Verification items for the finished model (mm, model axes). Face numbers are marked on the shaded views. Give positions to 0.01 mm unless a question says otherwise; leave off trailing zeros. Write each loop counter-clockwise with the first axis right and the second up, starting at its lowest first coordinate (ties: lowest second). Pieces come first, ordered by that corner, then holes. Notation, with made-up numbers: (-37.75, 1) -> (16.25, 1) arc R21 ccw to (16.25, 26) -> close; hole circle Ø6 at (13.25, 21.25). An arc over 180 degrees is marked (long way). Use one line per item in the form item = value. Start each with the question number.
(1) Section check A-A, the plane y = -50.8. Record the cut outline in (x, z).
(2) Depth check by flat-ended pin: pin 1 Ø2 at (y, z) = (-23, -80) entering from -X; pin 2 Ø10 at (x, y) = (-141, -20.5) entering from +Z; pin 3 Ø12.5 at (x, y) = (169, -68.5) entering from -Z. Enter the tip coordinate at first touch or a pass-through.
(3) Scan lines: L1, parallel to Z at x = -89, y = -24.5; L2, parallel to X at y = -82, z = -135; L3, parallel to X at y = -45, z = 368.5. Record each from-to range of solid material in increasing order.
(4) Section check B-B, the plane z = -79.5. Record the cut outline in (x, y), plus the area to 3 significant figures.
(5) Release check for a two-part mould opening along Z. For the marked faces 1, 2 and 3 record: pulls with the +Z half, pulls with the -Z half, needs draft (parallel to the pull), parting line crosses it, or undercut.
from build123d import *

# Parameters (mm, degrees)
F0_W        = 406.4
F0_H        = 635
F1_DEPTH    = 101.6
F2_W        = 129.6282266226
F2_H        = 559.1529050058
F2_W_2      = 230.7462543249
F2_H_2      = 486.9312153578
F3_DEPTH    = 127
F4_T1_DEPTH = 482.5995000003
F5_R        = 25.4
F6_R        = 25.4
F7_DEPTH    = 406.4
F8_R        = 6.35
F9_R        = 12.7
F10_DEPTH   = 25.4


# Not quite as in the source:
# - a fillet or chamfer that OpenCascade refuses, or shapes differently, is made with other operations: its cross-section is extruded or revolved along the edge and cut away or added
# - a feature names something its author has since deleted; it is built from what else it names


with BuildPart() as f1:
    # F0 (on Front) → F1 (new body)
    with BuildSketch(Plane.XZ):
        with Locations((-4.243819043, 96.6177646602)):
            Rectangle(F0_W, F0_H)
    extrude(amount=F1_DEPTH)

    # F2 (on face) → F3 (cut)
    with BuildSketch(Plane.XZ.offset(101.6)):
        with Locations((-234.1579323543, -322.6586878427)):
            Rectangle(F2_W, F2_H)
        with Locations((276.2293081194, -286.5478430187)):
            Rectangle(F2_W_2, F2_H_2)
    extrude(amount=-F3_DEPTH, mode=Mode.SUBTRACT)

    # F4: fillet of radius 76.2 on 2 edges, made by hand

    # F4_s2 → F4_t1 (cut)
    with BuildSketch(Plane.XZ.offset(-190.4997500002)):
        with BuildLine():
            ThreePointArc((198.956280957, 337.9178646602), (176.6378176834, 391.7994013866), (122.756280957, 414.1178646602))
            Line((122.756280957, 414.1178646602), (122.756280957, 415.6418646602))
            Line((122.756280957, 415.6418646602), (200.480180957, 415.6417646602))
            Line((200.480180957, 415.6417646602), (200.480280957, 337.9178646602))
            Line((200.480280957, 337.9178646602), (198.956280957, 337.9178646602))
        make_face()
        with BuildLine():
            ThreePointArc((-131.243919043, 414.1178646602), (-185.1254557695, 391.7994013866), (-207.443919043, 337.9178646602))
            Line((-207.443919043, 337.9178646602), (-208.967919043, 337.9178646602))
            Line((-208.967919043, 337.9178646602), (-208.967819043, 415.6417646602))
            Line((-208.967819043, 415.6417646602), (-131.243919043, 415.6418646602))
            Line((-131.243919043, 415.6418646602), (-131.243919043, 414.1178646602))
        make_face()
    extrude(amount=F4_T1_DEPTH, mode=Mode.SUBTRACT)

    # F5
    f5_edges = [f1.edges().sort_by_distance(p)[0] for p in [
        (198.956181, 0, 147.47954),
        (176.637818, 0, 391.799401),
        (-4.243819, 0, 414.117765),
        (-185.125456, 0, 391.799401),
        (-207.443819, 0, 147.47954),
    ]]
    fillet(f5_edges, radius=F5_R)

    # F6 (on face) → F7 (join)
    with BuildSketch(Plane.YZ.offset(198.956180957)):
        with Locations((-50.8, -119.2822353398)):
            Circle(F6_R)
    extrude(amount=-F7_DEPTH)

    # F8
    f8_edges = [f1.edges().sort_by_distance(p)[0] for p in [
        (-207.443819, -76.2, -119.282235),
        (198.956181, -76.2, -119.282235),
    ]]
    fillet(f8_edges, radius=F8_R)

    # F9
    f9_edges = [f1.edges().sort_by_distance(p)[0] for p in [
        (-169.343819, 0, -131.982235),
        (-175.693819, 0, -43.082235),
        (-200.004331, -7.439488, -43.082235),
        (-207.443819, -63.5, -43.082235),
        (160.856181, 0, -131.982235),
        (167.206181, 0, -43.082235),
        (191.516693, -7.439488, -43.082235),
        (198.956181, -63.5, -43.082235),
    ]]
    fillet(f9_edges, radius=F9_R)

    # F2 (on face) → F10 (cut)
    with BuildSketch(Plane.XZ.offset(101.6)):
        with Locations((-234.1579323543, -322.6586878427)):
            Rectangle(F2_W, F2_H)
        with Locations((276.2293081194, -286.5478430187)):
            Rectangle(F2_W_2, F2_H_2)
    extrude(amount=-F10_DEPTH, mode=Mode.SUBTRACT)


solid = f1.part
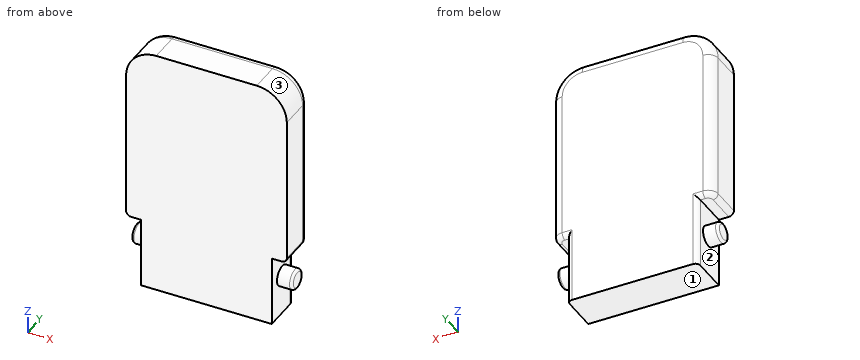
Completed:
q1.outline = (-207.44, -138.33) arc R6.35 ccw to (-201.09, -144.68) -> (-169.34, -144.68) -> (-169.34, -220.88) -> (160.86, -220.88) -> (160.86, -144.68) -> (192.61, -144.68) arc R6.35 ccw to (198.96, -138.33) -> (198.96, -100.23) arc R6.35 ccw to (192.61, -93.88) -> (160.86, -93.88) -> (160.86, -43.08) -> (186.26, -43.08) arc R12.7 ccw to (198.96, -30.38) -> (198.96, 338.04) arc R76.2 ccw to (122.88, 414.12) -> (-131.37, 414.12) arc R76.2 ccw to (-207.44, 338.04) -> (-207.44, -30.38) arc R12.7 ccw to (-194.74, -43.08) -> (-169.34, -43.08) -> (-169.34, -93.88) -> (-201.09, -93.88) arc R6.35 ccw to (-207.44, -100.23) -> close
q2.pin_1 = -169.34
q2.pin_2 = 413.83
q2.pin_3 = -141.96
q3.L1 = -220.88 to 414.1
q3.L2 = -169.34 to 160.86
q3.L3 = -201.04 to 192.55
q4.outline = (-169.34, -101.6) -> (160.86, -101.6) -> (160.86, -12.7) arc R12.7 ccw to (148.16, 0) -> (-156.64, 0) arc R12.7 ccw to (-169.34, -12.7) -> close
q4.area = 33,500 mm²
q5.face_1 = pulls with the -Z half
q5.face_2 = undercut
q5.face_3 = pulls with the +Z half
